Work out the finished part from the listing and answer in its coordinate system (mm). Face numbers are marked on the shaded views. A direction names the side the tool comes from. Round coordinates to 2 decimals unless told otherwise and drop trailing zeros. Order: outer loops, then holes, each group sorted by start corner. A loop starts at its lowest first (then second) coordinate and runs counter-clockwise, first axis right, second up. Notation, with made-up numbers: (71, 23.25) -> (120, 23.25) arc R26 cw to (120, 41.25) -> close; hole circle Ø8 at (-30, 55). An arc over 180 degrees is marked (long way). Use a Markdown table: item, result. Add a question column.
Item 1: Flat-ended cylindrical pins translate along their axes: P1, Ø22.5, axis at x = -33.59, z = 46.24, coming from the -Y side; P2, Ø4, axis at y = 6.5, z = -13.5, coming from the -X side; P3, Ø6, axis at x = -33.5, z = -88, coming from the +Y side; P4, Ø7.5, axis at x = 90.5, z = -52.25, coming from the -Y side. Find the tip coordinate at first contact, or state that the pin passes through.
Item 2: A tool of negligible diameter and unlimited length cuts with its end or side. For the marked faces 1 and 2, from which of +Z, -Z, +X, -X, +Y, -Y can it reach the whole face along a straight path? Write none if from no direction.
Item 3: For a pull along X with two mould halves and no side action, classify the marked faces 3 and 4 as +X half, -X half, draft (parallel to the pull), parting line (faces both ways), or undercut.
Item 4: A cutting plane is placed at B-B, the plane y = 2.5. Give the number of separate pieces and of enclosed holes in the cut face, plus the area to 3 significant figures.
Item 5: A cutting plane is placed at C-C, the plane x = 104.5. Determine the outline of the cut face in (y, z), plus the area to 3 significant figures.
Item 6: A cutting plane is placed at A-A, the plane z = -104.5. Determine the outline of the cut face in (x, y), plus the area to 3 significant figures.
Item 7: Find the intervals of material crossed by L1, parallel to Y at x = -56, z = 42.5; L2, parallel to Y at x = -38, z = -1; L3, parallel to X at y = 4.25, z = -98.5, in increasing order. Write a range as [from, to].
from build123d import *

# Parameters (mm, degrees)
SKETCH1_R           = 110.925
SKETCH1_R_2         = 3.2125
SKETCH1_R_3         = 98.075
BOSS_EXTRUDE1_DEPTH = 6.7
SKETCH2_R           = 72
SKETCH2_R_2         = 36.055
SKETCH2_R_3         = 7
BOSS_EXTRUDE3_DEPTH = 6.7
FILLET1_R           = 5
FILLET2_R           = 5
CHAMFER1_SIZE       = 3
CHAMFER2_SIZE       = 0.8
FILLET7_R           = 2.5
FILLET8_R           = 2.5


with BuildPart() as part:
    # Sketch1 → Boss-Extrude1 (new body)
    with BuildSketch(Plane(origin=(0, 0, 0), x_dir=(1, 0, 0), z_dir=(0, 1, 0))):
        with Locations(Location((0, 0, 0), (0, 0, 270))):
            Circle(SKETCH1_R)
        with Locations(Location((0, 104.5, 0), (0, 0, 270))):
            Circle(SKETCH1_R_2, mode=Mode.SUBTRACT)
        with Locations(Location((0, 0, 0), (0, 0, 270))):
            Circle(SKETCH1_R_3, mode=Mode.SUBTRACT)
        with Locations(Location((52.25, 90.499654695, 0), (0, 0, 270))):
            Circle(SKETCH1_R_2, mode=Mode.SUBTRACT)
        with Locations(Location((90.499654695, 52.25, 0), (0, 0, 270))):
            Circle(SKETCH1_R_2, mode=Mode.SUBTRACT)
        with Locations(Location((104.5, 0, 0), (0, 0, 270))):
            Circle(SKETCH1_R_2, mode=Mode.SUBTRACT)
        with Locations(Location((90.499654695, -52.25, 0), (0, 0, 270))):
            Circle(SKETCH1_R_2, mode=Mode.SUBTRACT)
        with Locations(Location((52.25, -90.499654695, 0), (0, 0, 270))):
            Circle(SKETCH1_R_2, mode=Mode.SUBTRACT)
        with Locations(Location((0, -104.5, 0), (0, 0, 270))):
            Circle(SKETCH1_R_2, mode=Mode.SUBTRACT)
        with Locations(Location((-52.25, -90.499654695, 0), (0, 0, 270))):
            Circle(SKETCH1_R_2, mode=Mode.SUBTRACT)
        with Locations(Location((-90.499654695, -52.25, 0), (0, 0, 270))):
            Circle(SKETCH1_R_2, mode=Mode.SUBTRACT)
        with Locations(Location((-104.5, 0, 0), (0, 0, 270))):
            Circle(SKETCH1_R_2, mode=Mode.SUBTRACT)
        with Locations(Location((-90.499654695, 52.25, 0), (0, 0, 270))):
            Circle(SKETCH1_R_2, mode=Mode.SUBTRACT)
        with Locations(Location((-52.25, 90.499654695, 0), (0, 0, 270))):
            Circle(SKETCH1_R_2, mode=Mode.SUBTRACT)
    extrude(amount=BOSS_EXTRUDE1_DEPTH)



with BuildPart() as body_2:
    # Sketch2 → Boss-Extrude3 (new body)
    with BuildSketch(Plane(origin=(0, 12.7, 0), x_dir=(1, 0, 0), z_dir=(0, 1, 0))):
        with Locations(Location((0, 0, 0), (0, 0, 270))):
            Circle(SKETCH2_R)
        with Locations(Location((0, 0, 0), (0, 0, 270))):
            Circle(SKETCH2_R_2, mode=Mode.SUBTRACT)
        with Locations(Location((0, 57.15, 0), (0, 0, 270))):
            Circle(SKETCH2_R_3, mode=Mode.SUBTRACT)
        with Locations(Location((54.352879906, 17.660321229, 0), (0, 0, 270))):
            Circle(SKETCH2_R_3, mode=Mode.SUBTRACT)
        with Locations(Location((33.591927169, -46.235321229, 0), (0, 0, 270))):
            Circle(SKETCH2_R_3, mode=Mode.SUBTRACT)
        with Locations(Location((-33.591927169, -46.235321229, 0), (0, 0, 270))):
            Circle(SKETCH2_R_3, mode=Mode.SUBTRACT)
        with Locations(Location((-54.352879906, 17.660321229, 0), (0, 0, 270))):
            Circle(SKETCH2_R_3, mode=Mode.SUBTRACT)
    extrude(amount=-BOSS_EXTRUDE3_DEPTH)


with BuildPart() as part_1:
    add(part.part)

    add(body_2.part)  # Sweep3 merges body 2
    # Sweep3: sweep along a curve in space
    with BuildLine() as sweep3_path:
        ThreePointArc((0, 6, 72), (50.911688245, 6, 50.911688245), (72, 6, 0))
        ThreePointArc((72, 6, 0), (50.911688245, 6, -50.911688245), (0, 6, -72))
        ThreePointArc((0, 6, -72), (-50.911688245, 6, -50.911688245), (-72, 6, 0))
        ThreePointArc((-72, 6, 0), (-50.911688245, 6, 50.911688245), (0, 6, 72))
    # Sketch4 → Sweep3 (sweep)
    with BuildSketch(Plane.XY):
        Polygon((72, 12.7), (98.075, 6.7), (98.075, 0), (72, 6), align=None)
    sweep(path=sweep3_path.line)

    # Fillet1
    fillet1_edges = [part_1.edges().sort_by_distance(p)[0] for p in [
        (50.911688245, 12.7, 50.911688245),
    ]]
    fillet(fillet1_edges, radius=FILLET1_R)

    # Fillet2
    fillet2_edges = [part_1.edges().sort_by_distance(p)[0] for p in [
        (69.349497565, 6.7, 69.349497565),
    ]]
    fillet(fillet2_edges, radius=FILLET2_R)

    # Chamfer1
    chamfer1_edges = [part_1.edges().sort_by_distance(p)[0] for p in [
        (0, 6, -36.055),
    ]]
    chamfer(chamfer1_edges, length=CHAMFER1_SIZE)

    # Chamfer2
    chamfer2_edges = [part_1.edges().sort_by_distance(p)[0] for p in [
        (-54.352879906, 6, -24.660321229),
        (-33.591927169, 6, 39.235321229),
        (33.591927169, 6, 39.235321229),
        (54.352879906, 6, -24.660321229),
        (0, 6, -64.15),
    ]]
    chamfer(chamfer2_edges, length=CHAMFER2_SIZE)

    # Fillet7
    fillet7_edges = [part_1.edges().sort_by_distance(p)[0] for p in [
        (50.911688245, 6, -50.911688245),
    ]]
    fillet(fillet7_edges, radius=FILLET7_R)

    # Fillet8
    fillet8_edges = [part_1.edges().sort_by_distance(p)[0] for p in [
        (69.349497565, 0, -69.349497565),
    ]]
    fillet(fillet8_edges, radius=FILLET8_R)


solid = part_1.part
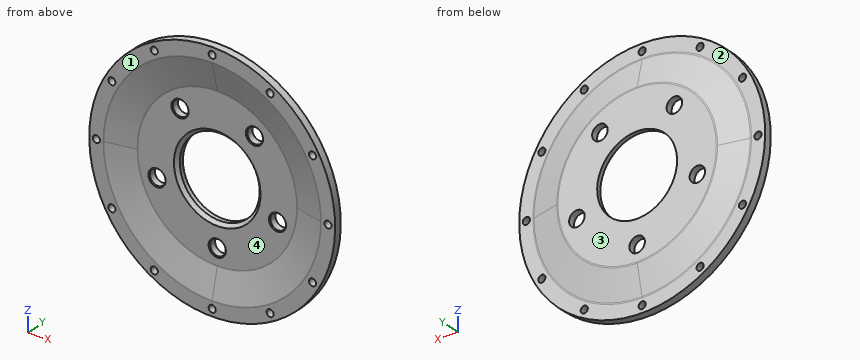
Reported:
| question | item | result |
|---|---|---|
| 1 | P1 | y = 6 |
| 1 | P2 | x = -110.33 |
| 1 | P3 | y = 8.29 |
| 1 | P4 | y = 0 |
| 2 | face 1 | +Z, -Z, +X, -X, -Y |
| 2 | face 2 | +Y |
| 3 | face 3 | draft |
| 3 | face 4 | undercut |
| 4 | separate pieces | 1 |
| 4 | enclosed holes | 13 |
| 4 | area | 14,400 mm² |
| 5 | outline | (0, -37.2) -> (6.7, -37.2) -> (6.7, -3.21) -> (0, -3.21) -> close; (0, 3.21) -> (6.7, 3.21) -> (6.7, 37.2) -> (0, 37.2) -> close |
| 5 | area | 455 mm² |
| 6 | outline | (-37.2, 0) -> (-3.21, 0) -> (-3.21, 6.7) -> (-37.2, 6.7) -> close; (3.21, 0) -> (37.2, 0) -> (37.2, 6.7) -> (3.21, 6.7) -> close |
| 6 | area | 455 mm² |
| 7 | L1 | [6, 12.7] |
| 7 | L2 | [7.04, 12.7] |
| 7 | L3 | [-51.01, 51.01] |
